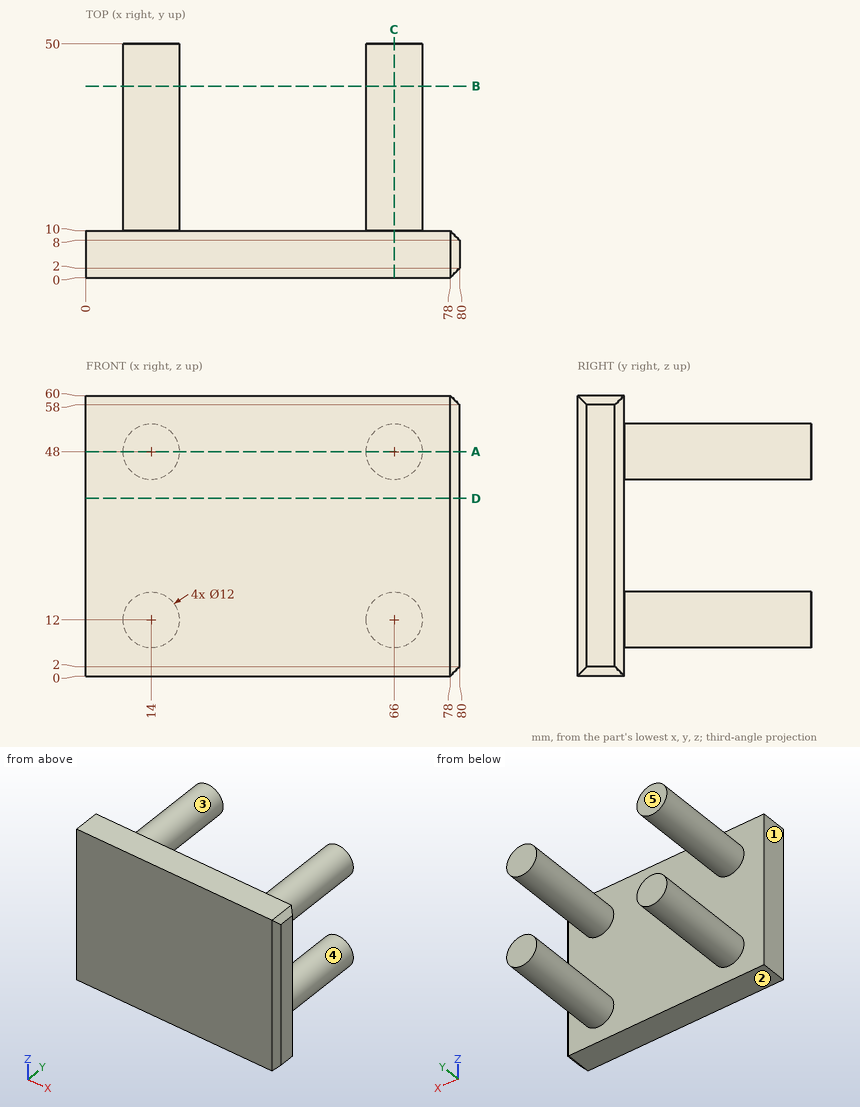
Here's the drawing with two shaded views (mm, measured from the low corner). I have some questions. A direction names the side the tool comes from. Give positions to 0.01 mm unless a question says otherwise; leave off trailing zeros. Loops run counter-clockwise (first coordinate to the right, second up) from the corner with the lowest first, then second, coordinate; pieces in that order, holes last. Notation, with made-up numbers: M 71.5,-29.5 L 107.5,-29.5 A26 cw 107.5,-6.5 Z; hole C 83,-38 d1. An arc over 180 degrees is marked long. One line per item, written item: value.
(1) Suppose I cut it at A-A on z = 48. List the corners of the cut face in (x, y) for me, plus the area to 3 significant figures.
Returned:
outline: M 0,0 L 78,0 L 80,2 L 80,8 L 78,10 L 72,10 L 72,50 L 60,50 L 60,10 L 20,10 L 20,50 L 8,50 L 8,10 L 0,10 Z
area: 1,760 mm^2
(2) Suppose I cut it at D-D on z = 38. List the corners of the cut face in (x, y) for me.
Returned:
outline: M 0,0 L 78,0 L 80,2 L 80,8 L 78,10 L 0,10 Z
(3) Will these pins go through, and if not, where does the flat tip stop? pin 1 (12 mm diameter, centred on x = 16, y = 29.5, fed in from -Z); pin 2 (1.5 mm diameter, centred on x = 11.5, y = 36.5, fed in from -Z).
Returned:
pin 1: z = 6
pin 2: z = 6.26
(4) Suppose I cut it at C-C on x = 66. List the corners of the cut face in (y, z) for me, plus the area to 3 significant figures.
Returned:
outline: M 0,0 L 10,0 L 10,6 L 50,6 L 50,18 L 10,18 L 10,42 L 50,42 L 50,54 L 10,54 L 10,60 L 0,60 Z
area: 1,560 mm^2
(5) Which directions (+Z, -Z, +X, -X, +Y, -Y) give clear straight access to the entire face, cutting with the end or side of a thin tool? Please do the marked faces 4 and 5.
Returned:
face 4: +Y
face 5: +Z, -Z, +X, -X, +Y
(6) I need wall thicknesses on line 1 (Y direction, x = 59, z = 26.5); line 2 (X direction, y = 31, z = 50); line 3 (Z direction, x = 62.5, y = 26). Which ranges of each line are inside material? Lowest first, please.
Returned:
line 1: 0 to 10
line 2: 8.34 to 19.66, 60.34 to 71.66
line 3: 7.13 to 16.87, 43.13 to 52.87
(7) Suppose I cut it at B-B on y = 41. List the corners of the cut face in (x, z) for me.
Returned:
outline: C 14,12 d12; C 14,48 d12; C 66,12 d12; C 66,48 d12
(8) We'd pull the mould along X, two halves only. Please class the marked faces 1, 2 and 3: released by +X, released by -X, zero draft, split by the parting line, or undercut.
Returned:
face 1: released by -X
face 2: zero draft
face 3: undercut
